Here's the drawing with two shaded views (mm, measured from the low corner). I have some questions. A direction names the side the tool comes from. Round coordinates to 2 decimals unless told otherwise and drop trailing zeros. Loops run counter-clockwise (first coordinate to the right, second up) from the corner with the lowest first, then second, coordinate; pieces in that order, holes last.
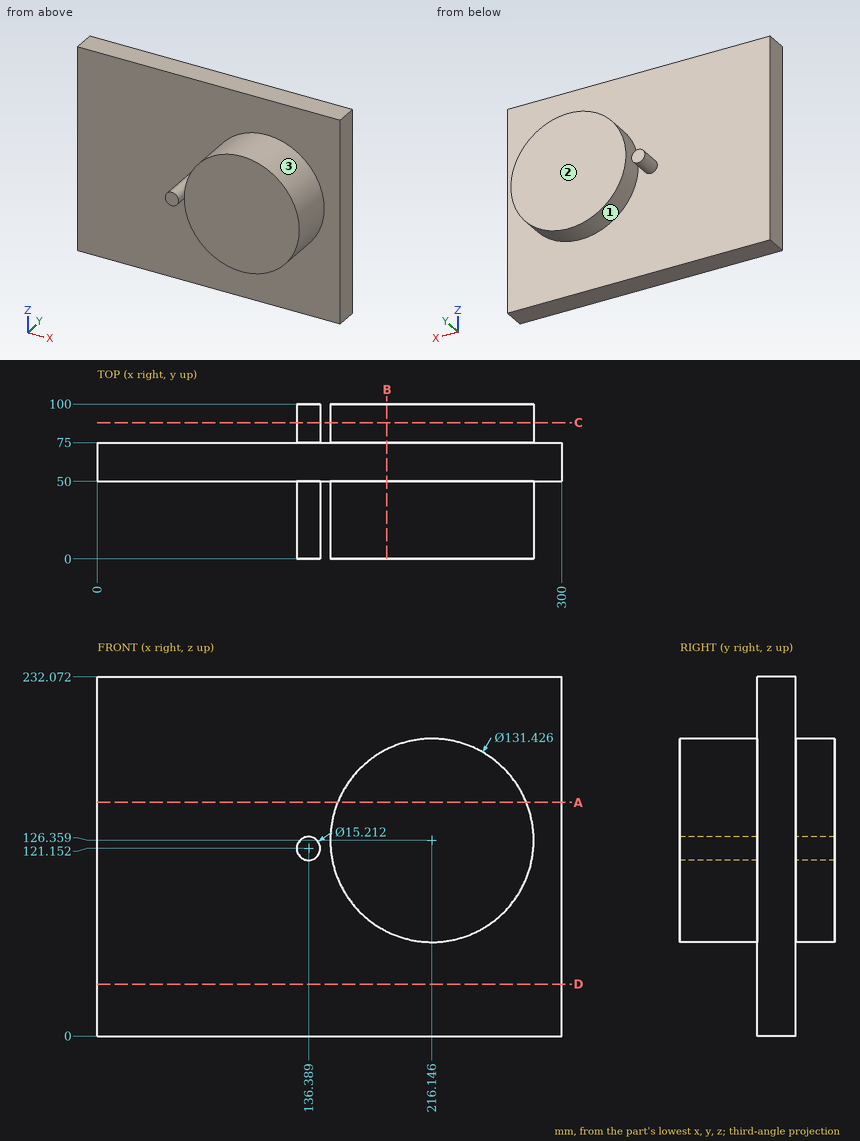
Item 1: If we section it at A-A, the plane z = 151: Please give me the cut outline in (x, y).
Results list:
outline: (0, 50) - (155.23, 50) - (155.23, 0) - (277.06, 0) - (277.06, 50) - (300, 50) - (300, 75) - (277.06, 75) - (277.06, 100) - (155.23, 100) - (155.23, 75) - (0, 75) - close
Item 2: If we section it at B-B, the plane x = 187: Please give me the cut outline in (y, z) (1 decimal).
Results list:
outline: (0, 67.5) - (50, 67.5) - (50, 0) - (75, 0) - (75, 67.5) - (100, 67.5) - (100, 185.3) - (75, 185.3) - (75, 232.1) - (50, 232.1) - (50, 185.3) - (0, 185.3) - close
Item 3: If we section it at D-D, the plane z = 33.5: Please give me the cut outline in (x, y), then the cut area to 3 significant figures.
Results list:
outline: (0, 50) - (300, 50) - (300, 75) - (0, 75) - close
area: 7,500 mm2
Item 4: If we section it at C-C, the plane y = 88: Please give me the cut outline in (x, z) (1 decimal).
Results list:
outline: circle Ø15.2 at (136.4, 121.2); circle Ø131.4 at (216.1, 126.4)
Item 5: Will these pins go through, and if not, where does the flat tip stop? pin 1 (8 mm diameter, centred on x = 210.5, y = 36.5, fed in from -Z); pin 2 (8 mm diameter, centred on x = 47, z = 86, fed in from +Y); pin 3 (3 mm diameter, centred on y = 77.5, z = 176.5, fed in from -X).
Results list:
pin 1: stops at z = 60.67
pin 2: stops at y = 75
pin 3: stops at x = 171.96
Item 6: If I drill on line 1 along Y through (x, z) = (135, 57); line 2 along Z through (x, y) = (169.5, 15.5) (1 decimal); line 3 along Z through (x, y) = (177.5, 81), over which ranges is the centre line in solid material (lowest first)?
Results list:
line 1: y = 50 to 75
line 2: z = 80.1 to 172.6
line 3: z = 73.21 to 179.51
Item 7: For the marked faces 1, 2 and 3, which set-ups out of +Z, -Z, +X, -X, +Y, -Y let a thin tool reach every point of the face, with its end or its side?
Results list:
face 1: +Y
face 2: +Z, -Z, +X, -X, +Y
face 3: -Y
